Source: CAD feature listing. Evaluate the final solid. Frame: model axes, mm. A direction names the side the tool comes from. Give positions to 0.01 mm unless a question says otherwise; leave off trailing zeros. Loops run counter-clockwise (first coordinate to the right, second up) from the corner with the lowest first, then second, coordinate; pieces in that order, holes last. Notation, with made-up numbers: M 34.5,83.25 L 43.5,83.25 A10 ccw 43.5,92.25 Z; hole C 58.5,76 d4. An arc over 180 degrees is marked long. Answer in a Markdown table with one row per item.
```python
from build123d import *

# Parameters (mm, degrees)
BOSS_EXTRU_1_DEPTH = 35


with BuildPart() as part:
    # Esquisse2 → Boss.-Extru.1 (new body)
    with BuildSketch(Plane.XY):
        with BuildLine():
            Line((0, 0), (-50, 0))
            ThreePointArc((-50, 0), (-67.5, 17.5), (-50, 35))
            Line((-50, 35), (0, 35))
            Line((0, 35), (0, 31))
            Line((0, 31), (-50, 31))
            ThreePointArc((-50, 31), (-63.5, 17.5), (-50, 4))
            Line((-50, 4), (0, 4))
            Line((0, 4), (0, 0))
        make_face()
    extrude(amount=BOSS_EXTRU_1_DEPTH)


solid = part.part
```
1) Material intervals for L1, parallel to Y at x = -18, z = 29.5; L2, parallel to X at y = 18, z = 6; L3, parallel to Y at x = -52, z = 9.5, sorted ascending.
Reply:
| item | result |
|---|---|
| L1 | y = 0 to 4, 31 to 35 |
| L2 | x = -67.49 to -63.49 |
| L3 | y = 0.11 to 4.15, 30.85 to 34.89 |
2) Section C-C, the plane y = 17.5. Return loops of the section in (x, z).
Reply:
| item | result |
|---|---|
| outline | M -67.5,0 L -63.5,0 L -63.5,35 L -67.5,35 Z |
3) Set-up query: faces 1 (the flat face through (-25, 31, 17)), 2 (the flat face through (-36, 3, 0)). Return all of +Z, -Z, +X, -X, +Y, -Y with unobstructed straight access to the full face (end or side cutting, diameter ignored); none if empty.
Reply:
| item | result |
|---|---|
| face 1 | +Z, -Z, +X |
| face 2 | -Z, +X, -X, +Y, -Y |
4) Section B-B, the plane z = 3. Return loops of the section in (x, y).
Reply:
| item | result |
|---|---|
| outline | M -50,0 L 0,0 L 0,4 L -50,4 A13.5 cw -50,31 L 0,31 L 0,35 L -50,35 A17.5 ccw Z |
5) Section D-D, the plane y = 32.5. Return loops of the section in (x, z), then the cut area to 3 significant figures.
Reply:
| item | result |
|---|---|
| outline | M -59.01,0 L 0,0 L 0,35 L -59.01,35 Z |
| area | 2,070 mm² |
6) Pin query (flat end, axial travel): pin 1 Ø1.5 at (y, z) = (26, 20) entering from +X. Return the tip coordinate at first contact, or that it passes through.
Reply:
| item | result |
|---|---|
| pin 1 | stops at x = -59.83 |
7) Section A-A, the plane x = -45.5. Return loops of the section in (y, z), then the cut area to 3 significant figures.
Reply:
| item | result |
|---|---|
| outline | M 0,0 L 4,0 L 4,35 L 0,35 Z; M 31,0 L 35,0 L 35,35 L 31,35 Z |
| area | 280 mm² |
